Could you check a few things on this model? Use its own coordinates, in mm. Face numbers are marked on the shaded views. Give positions to 0.01 mm unless a question says otherwise; leave off trailing zeros. Write each loop counter-clockwise with the first axis right and the second up, starting at its lowest first coordinate (ties: lowest second). Pieces come first, ordered by that corner, then holes. Notation, with made-up numbers: (49.25, -35.5) - (84.25, -35.5) arc R24 ccw to (84.25, -25.5) - close; hole circle Ø2 at (43.5, 35). An arc over 180 degrees is marked (long way). Answer as CSV lines item,"result". Start each with the question number.
Q1. Imagine slicing it at A-A on z = 0. List the corners of the cut face in (x, y) for me, and give its area (3 significant figures).
Q2. Imagine slicing it at B-B on y = 0. List the corners of the cut face in (x, z) for me, and give its area (3 significant figures).
Q3. If I drill on line 1 along Z through (x, y) = (7.75, 0); line 2 along X through (y, z) = (-4, -16.5); line 3 along Z through (x, y) = (1, 15), over which ranges is the centre line in solid material (lowest first)?
Q4. Will these pins go through, and if not, where does the flat tip stop? pin 1 Ø13 at (y, z) = (-1.5, 5.5) entering from +X; pin 2 Ø2 at (x, z) = (7, -5.5) entering from +Y; pin 3 Ø3.5 at (x, z) = (5.5, 0.5) entering from -Y; pin 4 Ø6 at (y, z) = (-18, 11) entering from +X.
Q5. Imagine slicing it at C-C on x = 6.5. List the corners of the cut face in (y, z) for me, and give its area (3 significant figures).
Q6. We'd pull the mould along Z, two halves only. Please class the marked faces 1, 2 and 3: pulls with the +Z half, pulls with the -Z half, needs draft (parallel to the pull), parting line crosses it, or undercut.
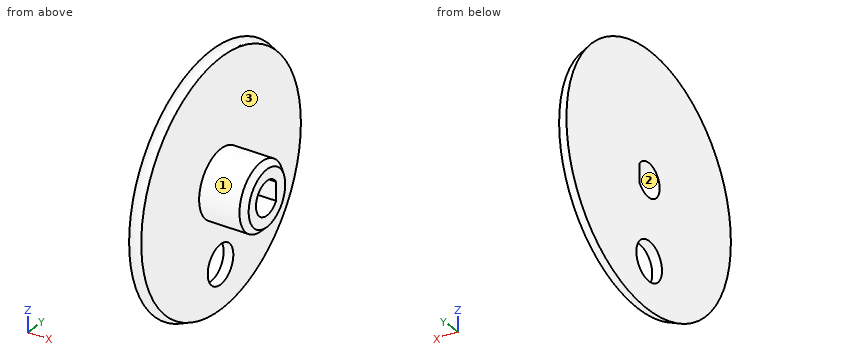
```python
from build123d import *

# Parameters (mm, degrees)
POCKET_DEPTH    = 10.001
CHAMFER_SIZE    = 1
SKETCH002_R     = 3.5
POCKET001_DEPTH = 5


with BuildPart() as part:
    # Sketch → Revolution (revolve)
    with BuildSketch(Plane.XY):
        with BuildLine():
            Line((0, 0), (0, 22.5))
            ThreePointArc((0, 22.5), (0.646447, 21.564586), (1.75, 21.838562))
            Line((1.75, 6), (1.75, 21.838562))
            Line((10, 6), (1.75, 6))
            Line((10, 0), (10, 6))
            Line((0, 0), (10, 0))
        make_face()
    revolve(axis=Axis((0, 0, 0), (1, 0, 0)))

    # Sketch001 (on Face5 of Revolution) → Pocket (cut, through all)
    with BuildSketch(Plane.YZ.offset(10)):
        with BuildLine():
            ThreePointArc((2.5, 1.658312), (-3, 0), (2.5, -1.658312))
            Line((2.5, 1.658312), (2.5, -1.658312))
        make_face()
    extrude(amount=-POCKET_DEPTH, mode=Mode.SUBTRACT)

    # Chamfer
    chamfer_edges = [part.edges().sort_by_distance(p)[0] for p in [
        (10, -6, 0),
    ]]
    chamfer(chamfer_edges, length=CHAMFER_SIZE)

    # Sketch002 (on Face6 of Chamfer) → Pocket001 (cut)
    with BuildSketch(Plane(origin=(0, 0, 0), x_dir=(0, -1, 0), z_dir=(-1, 0, 0))):
        with Locations((0.146868, -14)):
            Circle(SKETCH002_R)
    extrude(amount=-POCKET001_DEPTH, mode=Mode.SUBTRACT)


solid = part.part
```
Conclusion:
1,outline,"(0, -22.5) arc R1 cw to (1.75, -21.84) - (1.75, -6) - (9, -6) - (10, -5) - (10, -3) - (0, -3) - close; (0, 2.5) - (10, 2.5) - (10, 5) - (9, 6) - (1.75, 6) - (1.75, 21.84) arc R1 cw to (0, 22.5) - close"
1,area,"119 mm^2"
2,outline,"(0, -22.5) arc R1 cw to (1.75, -21.84) - (1.75, -17.5) - (0, -17.5) - close; (0, -10.5) - (1.75, -10.5) - (1.75, -6) - (9, -6) - (10, -5) - (10, -3) - (0, -3) - close; (0, 3) - (10, 3) - (10, 5) - (9, 6) - (1.75, 6) - (1.75, 21.84) arc R1 cw to (0, 22.5) - close"
2,area,"102 mm^2"
3,line 1,"-6 to -3, 3 to 6"
3,line 2,"0 to 1.75"
3,line 3,"-15.4 to 15.4"
4,pin 1,"x = 10"
4,pin 2,"y = 3.97"
4,pin 3,"y = -6"
4,pin 4,"x = 1.75"
5,outline,"circle Ø12 at (0, 0); hole (2.5, -1.66) - (2.5, 1.66) arc R3 ccw (long way) to start"
5,area,"85.9 mm^2"
6,face 1,"parting line crosses it"
6,face 2,"undercut"
6,face 3,"needs draft"
